Geometry: final body of the model. Coordinates: model frame, mm. Face numbers are marked on the shaded views. A direction names the side the tool comes from. Give positions to 0.01 mm unless a question says otherwise; leave off trailing zeros. Order: outer loops, then holes, each group sorted by start corner. A loop starts at its lowest first (then second) coordinate and runs counter-clockwise, first axis right, second up. Notation, with made-up numbers: (46, 89) -> (88, 89) arc R20 ccw to (88, 122) -> close; hole circle Ø2 at (-31.5, 42). An arc over 180 degrees is marked (long way). One line per question, with ' | ' between items. Start each with the question number.
(1) Mould query, pull axis X, two halves, no side actions, for the marked faces 3 and 4. Classes: +X half, -X half, draft (parallel to the pull), parting line (faces both ways), or undercut.
(2) Set-up query: the marked faces 1 and 2. Return all of +Z, -Z, +X, -X, +Y, -Y with unobstructed straight access to the full face (end or side cutting, diameter ignored); none if empty.
(3) Section A-A (y = -106.5). Return loops of the section in (x, z), then the cut area to 3 significant figures.
(4) Ray query, L1, parallel to X at y = -171, z = 8.75; L2, parallel to X at y = -48, z = 9; L3, parallel to X at y = -112, z = 9.5. Return the intervals inside material, ascending.
(5) Section B-B (z = 4). State how many separate pieces and enclosed holes the cut face has, then the cut area to 3 significant figures.
(6) First-contact query: pin 1 Ø6 at (y, z) = (-102.5, 5.5) entering from +X; pin 2 Ø3 at (y, z) = (-128, 3) entering from +X; pin 3 Ø5 at (x, z) = (3, 4) entering from -Y. Flat tips, straight axial feed; report the tip coordinate or a pass-through.
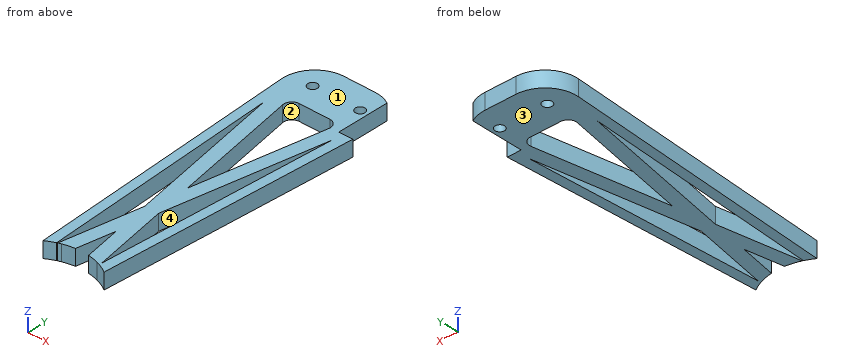
```python
from build123d import *

# Parameters (mm, degrees)
SKETCH1_R           = 3
BOSS_EXTRUDE2_DEPTH = 10
FILLET1_R           = 20
FILLET2_R           = 20
CUT_EXTRUDE1_START  = -10
CUT_EXTRUDE1_DEPTH  = 10
FILLET3_R           = 5
CUT_EXTRUDE5_START  = -10
SKETCH5_W           = 12
SKETCH5_H           = 10
CUT_EXTRUDE5_DEPTH  = 10


with BuildPart() as part:
    # Sketch1 → Boss-Extrude2 (new body)
    with BuildSketch(Plane.XY):
        with BuildLine():
            Line((-30, 15.770412854), (-30, 0))
            Line((-30, 0), (-17.5, -210))
            ThreePointArc((-17.5, -210), (0, -227.5), (17.5, -210))
            Line((17.5, -210), (30, 0))
            Line((30, 0), (30, 15.770412854))
            Line((30, 15.770412854), (-30, 15.770412854))
        make_face()
        with Locations((-15, 0)):
            Circle(SKETCH1_R, mode=Mode.SUBTRACT)
        with Locations((15, 0)):
            Circle(SKETCH1_R, mode=Mode.SUBTRACT)
        Polygon((0, -205), (6, -205), (6, -215), (-6, -215), (-6, -205), align=None, mode=Mode.SUBTRACT)
    extrude(amount=BOSS_EXTRUDE2_DEPTH)

    # Fillet1
    fillet1_edges = [part.edges().sort_by_distance(p)[0] for p in [
        (-30, 15.770412854, 5),
    ]]
    fillet(fillet1_edges, radius=FILLET1_R)

    # Fillet2
    fillet2_edges = [part.edges().sort_by_distance(p)[0] for p in [
        (30, 15.770412854, 5),
    ]]
    fillet(fillet2_edges, radius=FILLET2_R)

    # Sketch4 → Cut-Extrude1 (cut)
    with BuildSketch(Plane.XY.offset(10).offset(CUT_EXTRUDE1_START)):
        Polygon((-15.651797422, -15), (0.190220551, -102.160979768), (15.643622882, -15), (15, -15), align=None)
        Polygon((-22.473027071, -25.6531452), (-13.367328465, -178.628881795), (-4.134156204, -126.551525408), align=None)
        Polygon((22.230419841, -27.161313899), (4.615986353, -126.511039477), (13.430162671, -175.005634359), align=None)
        with BuildLine():
            Line((0.291609598, -150.901585116), (-7.372445375, -194.128735111))
            ThreePointArc((-7.372445375, -194.128735111), (0.476576628, -192.506490497), (8.225632191, -194.553674383))
            Line((8.225632191, -194.553674383), (0.291609598, -150.901585116))
        make_face()
    extrude(amount=CUT_EXTRUDE1_DEPTH, mode=Mode.SUBTRACT)

    # Fillet3
    fillet3_edges = [part.edges().sort_by_distance(p)[0] for p in [
        (8.225632191, -194.553674383, 5),
        (-7.372445375, -194.128735111, 5),
        (-15.651797422, -15, 5),
        (15.643622882, -15, 5),
    ]]
    fillet(fillet3_edges, radius=FILLET3_R)

    # Sketch5 → Cut-Extrude5 (cut)
    # profile 1 of 10: a face of its own
    with BuildSketch(Plane.XY.offset(10).offset(CUT_EXTRUDE5_START)):
        with BuildLine():
            Line((29.260488635, 0), (20, 0))
            Line((20, 0), (20, -20))
            Line((20, -20), (28.80952381, -20))
            Line((28.80952381, -20), (29.677502384, -5.417959945))
            ThreePointArc((29.677502384, -5.417959945), (29.653859351, -2.694751229), (29.260488635, 0))
        make_face()
    # profile 2 of 10: a face of its own
    with BuildSketch(Plane.XY.offset(10).offset(CUT_EXTRUDE5_START)):
        with BuildLine():
            Line((20, 12.921923742), (20, 0))
            Line((20, 0), (29.260488635, 0))
            ThreePointArc((29.260488635, 0), (25.96931496, 7.420606017), (20, 12.921923742))
        make_face()
    # profile 3 of 10: a face of its own
    with BuildSketch(Plane.XY.offset(10).offset(CUT_EXTRUDE5_START)):
        with BuildLine():
            Line((4.816305425, -175.795946561), (11.228656567, -175.795946561))
            ThreePointArc((11.228656567, -175.795946561), (7.921392788, -174.882318751), (4.542172021, -174.287695771))
            Line((4.542172021, -174.287695771), (4.816305425, -175.795946561))
        make_face()
    # profile 4 of 10: a face of its own
    with BuildSketch(Plane.XY.offset(10).offset(CUT_EXTRUDE5_START)):
        with BuildLine():
            ThreePointArc((19.308563513, -179.61613298), (15.387621929, -177.454323), (11.228656567, -175.795946561))
            Line((11.228656567, -175.795946561), (4.816305425, -175.795946561))
            Line((4.816305425, -175.795946561), (4.879901452, -176.145844664))
            ThreePointArc((4.879901452, -176.145844664), (12.347146855, -178.102269105), (19.185515511, -181.683339422))
            Line((19.185515511, -181.683339422), (19.308563513, -179.61613298))
        make_face()
    # profile 5 of 10: a face of its own
    with BuildSketch(Plane.XY.offset(10).offset(CUT_EXTRUDE5_START)):
        with BuildLine():
            Line((18.887385797, -186.691918617), (19.185515511, -181.683339422))
            ThreePointArc((19.185515511, -181.683339422), (12.347146855, -178.102269105), (4.879901452, -176.145844664))
            Line((4.879901452, -176.145844664), (5.679005105, -180.54242201))
            ThreePointArc((5.679005105, -180.54242201), (12.662186526, -182.803142969), (18.887385797, -186.691918617))
        make_face()
    # profile 6 of 10: a face of its own
    with BuildSketch(Plane.XY.offset(10).offset(CUT_EXTRUDE5_START)):
        with BuildLine():
            Line((17.5, -210), (18.887385797, -186.691918617))
            ThreePointArc((18.887385797, -186.691918617), (12.662186526, -182.803142969), (5.679005105, -180.54242201))
            Line((5.679005105, -180.54242201), (6.795310384, -186.684206595))
            ThreePointArc((6.795310384, -186.684206595), (5.577551358, -190.939561161), (1.45903868, -192.560928748))
            ThreePointArc((1.45903868, -192.560928748), (0.292984986, -192.502452749), (-0.874372768, -192.521857299))
            ThreePointArc((-0.874372768, -192.521857299), (-4.874459747, -190.834989527), (-6.047413252, -186.655228912))
            Line((-6.047413252, -186.655228912), (-4.940068564, -180.409533248))
            ThreePointArc((-4.940068564, -180.409533248), (-12.320876057, -182.646828096), (-18.887385797, -186.691918617))
            Line((-18.887385797, -186.691918617), (-17.5, -210))
            ThreePointArc((-17.5, -210), (0, -227.5), (17.5, -210))
        make_face()
        with Locations((0, -210)):
            Rectangle(SKETCH5_W, SKETCH5_H, mode=Mode.SUBTRACT)
    # profile 7 of 10: a face of its own
    with BuildSketch(Plane.XY.offset(10).offset(CUT_EXTRUDE5_START)):
        with BuildLine():
            Line((-4.167269409, -176.050756454), (-4.122092315, -175.795946561))
            Line((-4.122092315, -175.795946561), (-11.228656567, -175.795946561))
            ThreePointArc((-11.228656567, -175.795946561), (-12.106175916, -176.096600396), (-12.975657802, -176.419763184))
            Line((-12.975657802, -176.419763184), (-13.345719148, -178.506999951))
            ThreePointArc((-13.345719148, -178.506999951), (-8.842198544, -176.958619935), (-4.167269409, -176.050756454))
        make_face()
    # profile 8 of 10: a face of its own
    with BuildSketch(Plane.XY.offset(10).offset(CUT_EXTRUDE5_START)):
        with BuildLine():
            Line((-4.122092315, -175.795946561), (-3.840092025, -174.205395752))
            ThreePointArc((-3.840092025, -174.205395752), (-7.576229867, -174.806240028), (-11.228656567, -175.795946561))
            Line((-11.228656567, -175.795946561), (-4.122092315, -175.795946561))
        make_face()
    # profile 9 of 10: a face of its own
    with BuildSketch(Plane.XY.offset(10).offset(CUT_EXTRUDE5_START)):
        with BuildLine():
            ThreePointArc((-13.486799408, -176.621769943), (-16.46588928, -177.986339006), (-19.308563513, -179.61613298))
            Line((-19.308563513, -179.61613298), (-19.185515511, -181.683339422))
            ThreePointArc((-19.185515511, -181.683339422), (-16.356398794, -179.96026814), (-13.373872309, -178.518945203))
            Line((-13.373872309, -178.518945203), (-13.486799408, -176.621769943))
        make_face()
    # profile 10 of 10: a face of its own
    with BuildSketch(Plane.XY.offset(10).offset(CUT_EXTRUDE5_START)):
        with BuildLine():
            Line((-4.940068564, -180.409533248), (-4.167269409, -176.050756454))
            ThreePointArc((-4.167269409, -176.050756454), (-8.842198544, -176.958619935), (-13.345719148, -178.506999951))
            Line((-13.345719148, -178.506999951), (-13.367328465, -178.628881795))
            Line((-13.367328465, -178.628881795), (-13.373872309, -178.518945203))
            ThreePointArc((-13.373872309, -178.518945203), (-16.356398794, -179.96026814), (-19.185515511, -181.683339422))
            Line((-19.185515511, -181.683339422), (-18.887385797, -186.691918617))
            ThreePointArc((-18.887385797, -186.691918617), (-12.320876057, -182.646828096), (-4.940068564, -180.409533248))
        make_face()
    extrude(amount=CUT_EXTRUDE5_DEPTH, mode=Mode.SUBTRACT)


solid = part.part
```
Response:
1) face 3: draft | face 4: undercut
2) face 1: +Z, +X, -X, +Y, -Y | face 2: +Z, -Z
3) outline: (-23.66, 0) -> (-17.66, 0) -> (-17.66, 10) -> (-23.66, 10) -> close; (-7.78, 0) -> (8.16, 0) -> (8.16, 10) -> (-7.78, 10) -> close; (17.51, 0) -> (23.66, 0) -> (23.66, 10) -> (17.51, 10) -> close | area: 281 mm^2
4) L1: x = -19.82 to -13.82, -12.01 to -3.27, 3.94 to 12.7, 13.67 to 19.82 | L2: x = -27.14 to -21.14, -18.41 to -9.65, 9.79 to 18.54, 20.99 to 27.14 | L3: x = -23.33 to -17.33, -6.78 to 7.19, 17.18 to 23.33
5) separate pieces: 1 | enclosed holes: 4 | area: 5,900 mm^2
6) pin 1: stops at x = 24.08 | pin 2: stops at x = 22.47 | pin 3: stops at y = -174.42
